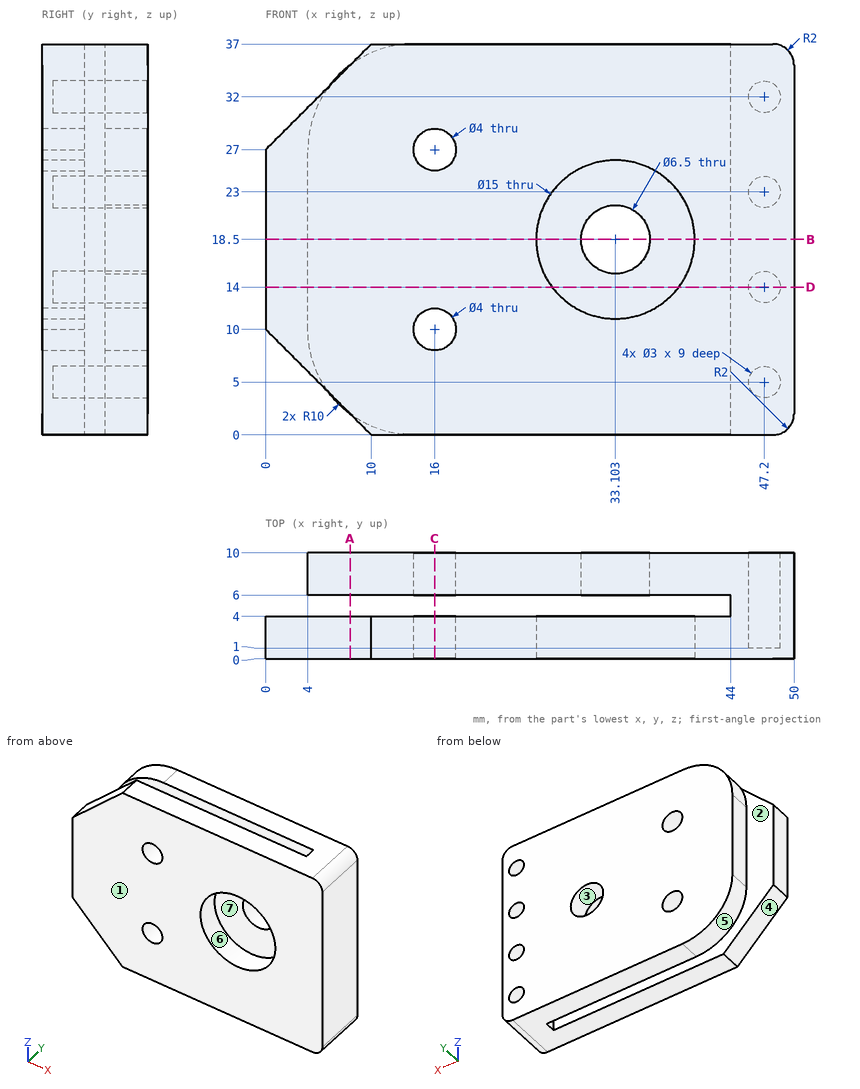
Input: dimensioned drawing with shaded views. Units: mm. Origin: part minimum x, y, z. A direction names the side the tool comes from. Coordinates: 2 decimals unless noted, no trailing zeros. Order: outer loops, then holes, each group sorted by start corner. A loop starts at its lowest first (then second) coordinate and runs counter-clockwise, first axis right, second up.
(1) Section query C-C (x = 16). Return the cut outline in (y, z).
(2) Section query A-A (x = 8). Return the cut outline in (y, z), plus the area to 3 significant figures.
(3) First-contact query: pin 1 (3.5 mm diameter, centred on x = 16, z = 27, fed in from +Y); pin 2 (2 mm diameter, centred on y = 5.5, z = 20, fed in from -X). Flat tips, straight axial feed; report the tip coordinate or a pass-through.
(4) Section query B-B (z = 18.5). Return the cut outline in (x, y).
(5) Draft query along Y for the marked faces 1, 2 and 3. Return one class per face: pulls with the +Y half, pulls with the -Y half, needs draft (parallel to the pull), parting line crosses it, or undercut.
(6) Section query D-D (z = 14). Return the cut outline in (x, y), plus the area to 3 significant figures.
(7) Access query for the marked faces 4, 5, 6 and 7. Directions: +Z, -Z, +X, -X, +Y, -Y. A direction counts if a zero-diameter tool reaches every point of the face in a straight line with its end or side. Return the directions, or none.
(8) Material intervals for probe 1 along Z at (x, y) = (47.2, 5); probe 2 along Y at (x, z) = (42, 6); probe 3 along Z at (x, y) = (17, 0.5), sorted ascending.
Solution:
1. outline: (0, 0) - (4, 0) - (4, 8) - (0, 8) - close; (0, 12) - (4, 12) - (4, 25) - (0, 25) - close; (0, 29) - (4, 29) - (4, 37) - (0, 37) - close; (6, 0) - (10, 0) - (10, 8) - (6, 8) - close; (6, 12) - (10, 12) - (10, 25) - (6, 25) - close; (6, 29) - (10, 29) - (10, 37) - (6, 37) - close
2. outline: (0, 2) - (4, 2) - (4, 35) - (0, 35) - close; (6, 2) - (10, 2) - (10, 35) - (6, 35) - close
2. area: 264 mm2
3. pin 1: passes through
3. pin 2: stops at x = 4
4. outline: (0, 0) - (25.6, 0) - (25.6, 4) - (0, 4) - close; (4, 6) - (29.85, 6) - (29.85, 10) - (4, 10) - close; (36.35, 6) - (44, 6) - (44, 4) - (40.6, 4) - (40.6, 0) - (50, 0) - (50, 10) - (36.35, 10) - close
5. face 1: pulls with the -Y half
5. face 2: undercut
5. face 3: needs draft
6. outline: (0, 0) - (27.1, 0) - (27.1, 4) - (0, 4) - close; (4, 6) - (44, 6) - (44, 4) - (39.1, 4) - (39.1, 0) - (50, 0) - (50, 10) - (48.7, 10) - (48.7, 1) - (45.7, 1) - (45.7, 10) - (4, 10) - close
6. area: 321 mm2
7. face 4: -Z, -X, -Y
7. face 5: -Z, -X, +Y
7. face 6: -Y
7. face 7: +Z, -Z, -X
8. probe 1: z = 0 to 3.5, 6.5 to 12.5, 15.5 to 21.5, 24.5 to 30.5, 33.5 to 37
8. probe 2: y = 0 to 4, 6 to 10
8. probe 3: z = 0 to 8.27, 11.73 to 25.27, 28.73 to 37
